Input: dimensioned drawing with shaded views. Units: mm. Origin: part minimum x, y, z. A direction names the side the tool comes from. Give positions to 0.01 mm unless a question says otherwise; leave off trailing zeros. Write each loop counter-clockwise with the first axis right and the second up, starting at its lowest first coordinate (ties: lowest second). Pieces come first, ordered by that corner, then holes.
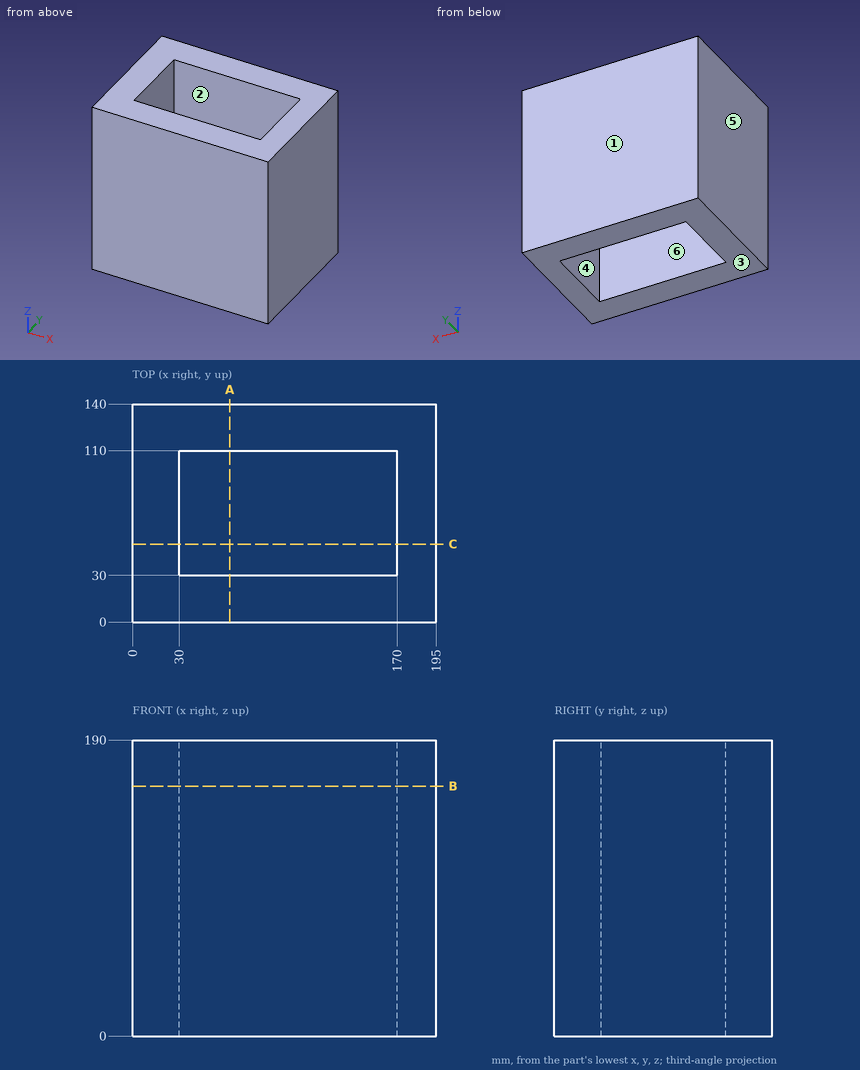
Item 1: Section A-A, the plane x = 62.5. Return the cut outline in (y, z), plus the area to 3 significant figures.
Found:
outline: (0, 0) - (30, 0) - (30, 190) - (0, 190) - close; (110, 0) - (140, 0) - (140, 190) - (110, 190) - close
area: 11,400 mm2
Item 2: Line query: L1, parallel to X at y = 49, z = 70; L2, parallel to Y at x = 122.5, z = 101. Output: solid intervals per line, ascending.
Found:
L1: x = 0 to 30, 170 to 195
L2: y = 0 to 30, 110 to 140
Item 3: Section C-C, the plane y = 50. Return the cut outline in (x, z), plus the area to 4 significant figures.
Found:
outline: (0, 0) - (30, 0) - (30, 190) - (0, 190) - close; (170, 0) - (195, 0) - (195, 190) - (170, 190) - close
area: 10,450 mm2
Item 4: Reachability of the marked faces 1 and 2 from +Z, -Z, +X, -X, +Y, -Y: full face, straight path, thin tool, end or side. Return the list, or none.
Found:
face 1: +Z, -Z, +X, -X, +Y
face 2: +Z, -Z
Item 5: Section B-B, the plane z = 160.5. Return the cut outline in (x, y).
Found:
outline: (0, 0) - (195, 0) - (195, 140) - (0, 140) - close; hole (30, 30) - (170, 30) - (170, 110) - (30, 110) - close
Item 6: Pull-direction query (X, two-part tool) for the marked faces 3, 4, 5 and 6; classes: +X half, -X half, draft (parallel to the pull), parting line (faces both ways), or undercut.
Found:
face 3: draft
face 4: undercut
face 5: -X half
face 6: undercut
